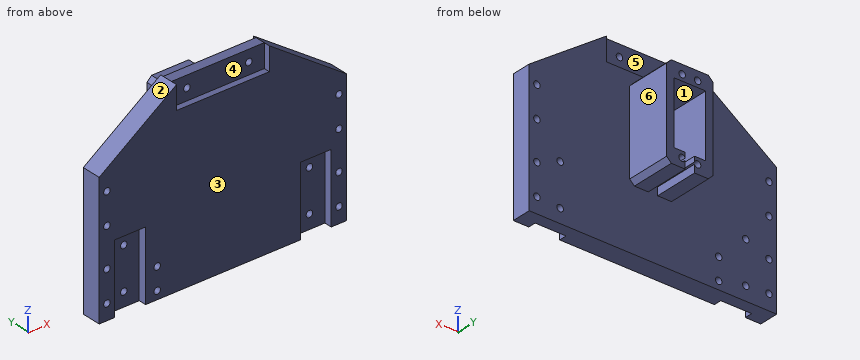
```python
from build123d import *

# Parameters (mm, degrees)
BOSS_EXTRUDE2_DEPTH = 12.5
SKETCH2_R           = 2.1
BOSS_EXTRUDE3_DEPTH = 29
SKETCH4_W           = 9
SKETCH4_H           = 3.5
CUT_EXTRUDE1_DEPTH  = 73
CHAMFER1_SIZE       = 3
SKETCH5_W           = 60
SKETCH5_H           = 15
SKETCH5_R           = 2.89755201
CUT_EXTRUDE2_DEPTH  = 4
SKETCH6_R           = 2.89755201
CUT_EXTRUDE3_DEPTH  = 26
SKETCH7_R           = 2.1
CUT_EXTRUDE4_DEPTH  = 26
SKETCH8_R           = 2.1
CUT_EXTRUDE5_DEPTH  = 26
SKETCH9_W           = 20
SKETCH9_H           = 45
CUT_EXTRUDE8_DEPTH  = 5
SKETCH10_W          = 1.5
SKETCH10_H          = 3.5
BOSS_EXTRUDE4_DEPTH = 9.75
SKETCH11_R          = 2.1
CUT_EXTRUDE9_DEPTH  = 22
SKETCH12_R          = 2.89755201
SKETCH12_R_2        = 2.1
BOSS_EXTRUDE6_DEPTH = 8.5
SKETCH13_W          = 1.5
SKETCH13_H          = 3.5
CUT_EXTRUDE10_DEPTH = 14.2
SKETCH14_W          = 60
SKETCH14_H          = 15
CUT_EXTRUDE11_DEPTH = 2
BOSS_EXTRUDE7_REACH = 43.5
SKETCH15_R          = 2.1


with BuildPart() as part:
    # Sketch1 → Boss-Extrude2 (new body)
    with BuildSketch(Plane(origin=(0, 0, 0), x_dir=(1, 0, 0), z_dir=(0, 1, 0))):
        Polygon((-80, -42.5), (-80, 42.5), (80, 42.5), (80, -42.5), (30, -77.5), (-30, -77.5), align=None)
    extrude(amount=BOSS_EXTRUDE2_DEPTH)

    # Sketch2 → Boss-Extrude3 (add)
    with BuildSketch(Plane(origin=(0, 12.5, 0), x_dir=(1, 0, 0), z_dir=(0, 1, 0))):
        with BuildLine():
            Line((10.25, -47.5), (-10.25, -47.5))
            Line((-10.25, -47.5), (-10.25, -7))
            Line((-10.25, -7), (-3, -7))
            Line((-3, -7), (-3, -3.640312424))
            ThreePointArc((-3, -3.640312424), (-7.1, -3), (-3, -2.359687576))
            Line((-3, -2.359687576), (-3, 2.75))
            Line((-3, 2.75), (-15, 2.75))
            Line((-15, 2.75), (-15, -57.25))
            Line((-15, -57.25), (15, -57.25))
            Line((15, -57.25), (15, 2.75))
            Line((15, 2.75), (3, 2.75))
            Line((3, 2.75), (3, -2.359687576))
            ThreePointArc((3, -2.359687576), (5.324037035, -0.925150608), (7.1, -3))
            ThreePointArc((7.1, -3), (5.324037035, -5.074849392), (3, -3.640312424))
            Line((3, -3.640312424), (3, -7))
            Line((3, -7), (10.25, -7))
            Line((10.25, -7), (10.25, -47.5))
        make_face()
        with Locations((-5, -51.5)):
            Circle(SKETCH2_R, mode=Mode.SUBTRACT)
        with Locations((5, -51.5)):
            Circle(SKETCH2_R, mode=Mode.SUBTRACT)
    extrude(amount=BOSS_EXTRUDE3_DEPTH)

    # Sketch4 → Cut-Extrude1 (cut)
    with BuildSketch(Plane.XY.offset(57.25)):
        with Locations((5, 35.75)):
            Rectangle(SKETCH4_W, SKETCH4_H)
        with Locations((-5, 35.75)):
            Rectangle(SKETCH4_W, SKETCH4_H)
    extrude(amount=-CUT_EXTRUDE1_DEPTH, mode=Mode.SUBTRACT)

    # Chamfer1
    chamfer1_edges = [part.edges().sort_by_distance(p)[0] for p in [
        (-15, 27, -2.75),
        (-15, 27, 57.25),
        (15, 27, 57.25),
        (15, 27, -2.75),
    ]]
    chamfer(chamfer1_edges, length=CHAMFER1_SIZE)

    # Sketch5 → Cut-Extrude2 (cut)
    with BuildSketch(Plane.XZ):
        with Locations((0, 70)):
            Rectangle(SKETCH5_W, SKETCH5_H)
        with Locations((-20, 70)):
            Circle(SKETCH5_R, mode=Mode.SUBTRACT)
        with Locations((20, 70)):
            Circle(SKETCH5_R, mode=Mode.SUBTRACT)
    extrude(amount=-CUT_EXTRUDE2_DEPTH, mode=Mode.SUBTRACT)

    # Sketch6 → Cut-Extrude3 (cut)
    with BuildSketch(Plane(origin=(0, 0, 0), x_dir=(-1, 0, 0), z_dir=(0, -1, 0))):
        with Locations((20, -70)):
            Circle(SKETCH6_R)
        with Locations((-20, -70)):
            Circle(SKETCH6_R)
    extrude(amount=-CUT_EXTRUDE3_DEPTH, mode=Mode.SUBTRACT)

    # Sketch7 → Cut-Extrude4 (cut)
    with BuildSketch(Plane(origin=(0, 12.5, 0), x_dir=(1, 0, 0), z_dir=(0, 1, 0))):
        with Locations((-75, 32.5)):
            Circle(SKETCH7_R)
        with Locations((-75, 12.5)):
            Circle(SKETCH7_R)
        with Locations((-75, -12.5)):
            Circle(SKETCH7_R)
        with Locations((-75, -32.5)):
            Circle(SKETCH7_R)
        with Locations((75, -32.5)):
            Circle(SKETCH7_R)
        with Locations((75, -12.5)):
            Circle(SKETCH7_R)
        with Locations((75, 12.5)):
            Circle(SKETCH7_R)
        with Locations((75, 32.5)):
            Circle(SKETCH7_R)
    extrude(amount=-CUT_EXTRUDE4_DEPTH, mode=Mode.SUBTRACT)

    # Sketch8 → Cut-Extrude5 (cut)
    with BuildSketch(Plane.XZ):
        with Locations((-60, -6.5)):
            Circle(SKETCH8_R)
        with Locations((-60, -33.5)):
            Circle(SKETCH8_R)
        with Locations((60, -6.5)):
            Circle(SKETCH8_R)
        with Locations((60, -33.5)):
            Circle(SKETCH8_R)
    extrude(amount=-CUT_EXTRUDE5_DEPTH, mode=Mode.SUBTRACT)

    # Sketch9 → Cut-Extrude8 (cut)
    with BuildSketch(Plane.XZ):
        with Locations((-60, -20)):
            Rectangle(SKETCH9_W, SKETCH9_H)
        with Locations((60, -20)):
            Rectangle(SKETCH9_W, SKETCH9_H)
    extrude(amount=-CUT_EXTRUDE8_DEPTH, mode=Mode.SUBTRACT)

    # Sketch10 → Boss-Extrude4 (add)
    with BuildSketch(Plane.XY.offset(57.25)):
        with Locations((0, 35.75)):
            Rectangle(SKETCH10_W, SKETCH10_H)
    extrude(amount=-BOSS_EXTRUDE4_DEPTH)

    # Sketch11 → Cut-Extrude9 (cut)
    with BuildSketch(Plane(origin=(0, 12.5, 0), x_dir=(1, 0, 0), z_dir=(0, 1, 0))):
        with Locations((-42.5, 37.25)):
            Circle(SKETCH11_R)
        with Locations((-42.5, 23.25)):
            Circle(SKETCH11_R)
    extrude(amount=-CUT_EXTRUDE9_DEPTH, mode=Mode.SUBTRACT)

    # Sketch12 → Boss-Extrude6 (add)
    with BuildSketch(Plane(origin=(0, 12.5, 0), x_dir=(1, 0, 0), z_dir=(0, 1, 0))):
        with Locations((-20, -70)):
            Circle(SKETCH12_R)
        with Locations((-20, -70)):
            Circle(SKETCH12_R_2, mode=Mode.SUBTRACT)
        with Locations((20, -70)):
            Circle(SKETCH12_R)
        with Locations((20, -70)):
            Circle(SKETCH12_R_2, mode=Mode.SUBTRACT)
    extrude(amount=-BOSS_EXTRUDE6_DEPTH)

    # Sketch13 → Cut-Extrude10 (cut)
    with BuildSketch(Plane.XY.offset(57.25)):
        with Locations((0, 35.75)):
            Rectangle(SKETCH13_W, SKETCH13_H)
    extrude(amount=-CUT_EXTRUDE10_DEPTH, mode=Mode.SUBTRACT)

    # Sketch14 → Cut-Extrude11 (cut)
    with BuildSketch(Plane(origin=(0, 12.5, 0), x_dir=(1, 0, 0), z_dir=(0, 1, 0))):
        with Locations((0, -70)):
            Rectangle(SKETCH14_W, SKETCH14_H)
    extrude(amount=-CUT_EXTRUDE11_DEPTH, mode=Mode.SUBTRACT)

    # Sketch15 → Boss-Extrude7 (add, up to next)
    with BuildSketch(Plane(origin=(0, 41.5, 0), x_dir=(1, 0, 0), z_dir=(0, 1, 0)), mode=Mode.PRIVATE) as boss_extrude7_sk1:
        Polygon((-12, -47.5), (-12, -57.25), (12, -57.25), (12, -47.5), (10.25, -47.5), (-10.25, -47.5), align=None)
        with Locations((-5, -51.5)):
            Circle(SKETCH15_R, mode=Mode.SUBTRACT)
        with Locations((5, -51.5)):
            Circle(SKETCH15_R, mode=Mode.SUBTRACT)
    boss_extrude7_tool1 = extrude(boss_extrude7_sk1.sketch, amount=-BOSS_EXTRUDE7_REACH, mode=Mode.PRIVATE) - part.part
    add(boss_extrude7_tool1.solids().sort_by_distance((0, 41.5, 52.492529))[0])
    # Sketch15 → Boss-Extrude7 (add, up to next)
    with BuildSketch(Plane(origin=(0, 41.5, 0), x_dir=(1, 0, 0), z_dir=(0, 1, 0)), mode=Mode.PRIVATE) as boss_extrude7_sk2:
        with BuildLine():
            Line((12, 2.75), (3, 2.75))
            Line((3, 2.75), (3, -2.359687576))
            ThreePointArc((3, -2.359687576), (5.324037035, -0.925150608), (7.1, -3))
            ThreePointArc((7.1, -3), (5.324037035, -5.074849392), (3, -3.640312424))
            Line((3, -3.640312424), (3, -7))
            Line((3, -7), (10.25, -7))
            Line((10.25, -7), (12.122605781, -7))
            Line((12.122605781, -7), (12.122605781, 2.627394219))
            Line((12.122605781, 2.627394219), (12, 2.75))
        make_face()
    boss_extrude7_tool2 = extrude(boss_extrude7_sk2.sketch, amount=-BOSS_EXTRUDE7_REACH, mode=Mode.PRIVATE) - part.part
    add(boss_extrude7_tool2.solids().sort_by_distance((8.027672, 41.5, 1.965211))[0])
    # Sketch15 → Boss-Extrude7 (add, up to next)
    with BuildSketch(Plane(origin=(0, 41.5, 0), x_dir=(1, 0, 0), z_dir=(0, 1, 0)), mode=Mode.PRIVATE) as boss_extrude7_sk3:
        with BuildLine():
            Line((-3, 2.75), (-12, 2.75))
            Line((-12, 2.75), (-12, -7))
            Line((-12, -7), (-10.25, -7))
            Line((-10.25, -7), (-3, -7))
            Line((-3, -7), (-3, -3.640312424))
            ThreePointArc((-3, -3.640312424), (-7.1, -3), (-3, -2.359687576))
            Line((-3, -2.359687576), (-3, 2.75))
        make_face()
    boss_extrude7_tool3 = extrude(boss_extrude7_sk3.sketch, amount=-BOSS_EXTRUDE7_REACH, mode=Mode.PRIVATE) - part.part
    add(boss_extrude7_tool3.solids().sort_by_distance((-7.962908, 41.5, 1.962154))[0])


solid = part.part
```
Could you check a few things on this model? Use its own coordinates, in mm. Face numbers are marked on the shaded views. A direction names the side the tool comes from. Coordinates: 2 decimals unless noted, no trailing zeros. Order: outer loops, then holes, each group sorted by start corner. A loop starts at its lowest first (then second) coordinate and runs counter-clockwise, first axis right, second up. Notation, with made-up numbers: M 35.25,72.5 L 60.25,72.5 A27 ccw 60.25,111.5 Z; hole C 88.5,13.25 d1. An arc over 180 degrees is marked long. Use a Markdown table: item, result. Add a question column.
Q1. I want a section at A-A on z = 32.5. List the corners of the cut face in (x, y) for me, then the cut area to 3 significant figures.
Q2. I'm going to push flat-ended pins straight in: pin 1 (5 mm diameter, centred on y = 23, z = 19, fed in from +X); pin 2 (5.5 mm diameter, centred on x = 75, z = 32.5, fed in from +Y); pin 3 (1.7 mm diameter, centred on y = 23.5, z = 5, fed in from -X). Where does each tip first touch, or does it pass through?
Q3. If I drill on L1, parallel to Z at x = 5, y = 20.5; L2, parallel to X at y = 39.6, z = 51.5; L3, parallel to X at y = 3, z = -37, over which ranges is the centre line in solid material (lowest first)?
Q4. Which directions (+Z, -Z, +X, -X, +Y, -Y) give clear straight access to the entire face, cutting with the end or side of a thin tool? Please do the marked faces 4, 5 and 6.
Q5. I want a section at D-D on z = 20.5. List the corners of the cut face in (x, y) for me, then the cut area to 3 significant figures.
Q6. I want a section at B-B on y = 24.5. List the corners of the cut face in (x, z) for me, then the cut area to 3 significant figures.
Q7. I want a section at C-C on x = 24. List the corners of the cut face in (y, z) for me.
Q8. We'd pull the mould along Z, two halves only. Please class the marked faces 1, 2 and 3: pulls with the +Z half, pulls with the -Z half, needs draft (parallel to the pull), parting line crosses it, or undercut.
Checked values:
| question | item | result |
|---|---|---|
| 1 | outline | M -80,0 L -77.1,0 L -77.1,12.5 L -80,12.5 Z; M -72.9,0 L 72.9,0 L 72.9,12.5 L 15,12.5 L 15,41.5 L 10.25,41.5 L 10.25,12.5 L -10.25,12.5 L -10.25,41.5 L -15,41.5 L -15,12.5 L -72.9,12.5 Z; M 77.1,0 L 80,0 L 80,12.5 L 77.1,12.5 Z |
| 1 | area | 2,170 mm² |
| 2 | pin 1 | x = 15 |
| 2 | pin 2 | y = 12.5 |
| 2 | pin 3 | x = -15 |
| 3 | L1 | -2.75 to 0.9, 5.1 to 7, 47.5 to 49.4, 53.6 to 57.25 |
| 3 | L2 | -15 to -7.1, -2.9 to 2.9, 7.1 to 15 |
| 3 | L3 | -80 to -70, -50 to -44.59, -40.41 to 50, 70 to 80 |
| 4 | face 4 | +Z, -Y |
| 4 | face 5 | +Z, +Y |
| 4 | face 6 | +Z, -Z, +X, +Y |
| 5 | outline | M -80,0 L 80,0 L 80,12.5 L 15,12.5 L 15,41.5 L 10.25,41.5 L 10.25,12.5 L -10.25,12.5 L -10.25,41.5 L -15,41.5 L -15,12.5 L -80,12.5 Z |
| 5 | area | 2,280 mm² |
| 6 | outline | M -15,0.25 L -12,-2.75 L -3,-2.75 L -3,2.36 A2.1 cw long -3,3.64 L -3,7 L -10.25,7 L -10.25,47.5 L 10.25,47.5 L 10.25,7 L 3,7 L 3,3.64 A2.1 cw long 3,2.36 L 3,-2.75 L 12,-2.75 L 15,0.25 L 15,54.25 L 12,57.25 L -12,57.25 L -15,54.25 Z; hole C -5,51.5 d4.2; hole C 5,51.5 d4.2 |
| 6 | area | 838 mm² |
| 7 | outline | M 0,-42.5 L 12.5,-42.5 L 12.5,62.5 L 10.5,62.5 L 10.5,77.5 L 4,77.5 L 4,62.5 L 0,62.5 Z |
| 8 | face 1 | undercut |
| 8 | face 2 | pulls with the +Z half |
| 8 | face 3 | needs draft |
